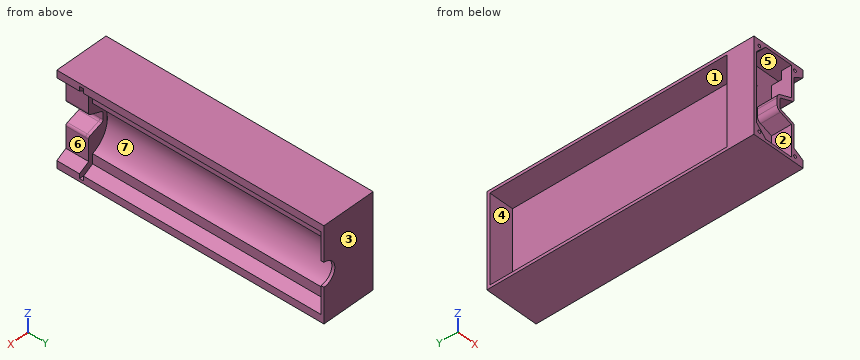
```python
from build123d import *

# Parameters (mm, degrees)
EXTRUDE_1_DEPTH     = 96
EXTRUDE_2_DEPTH     = 1.2
SKETCH_3_R          = 1.6
SKETCH_3_R_2        = 0.6
EXTRUDE_3_DEPTH     = 1.6
SKETCH_4_R          = 0.6
SKETCH_4_R_2        = 1.6
EXTRUDE_4_DEPTH     = 1.2
FILLET_1_R          = 1
SKETCH_5_R          = 1.5
CUT_EXTRUDE_1_DEPTH = 2
SKETCH_6_R          = 1.5
CUT_EXTRUDE_2_DEPTH = 2
EXTRUDE_START       = 8
EXTRUDE_6_DEPTH     = 8
SKETCH_10_R         = 0.6
EXTRUDE_7_DEPTH     = 4


with BuildPart() as part:
    # Эскиз1 → Бобышка-Вытянуть1 (new body)
    with BuildSketch(Plane(origin=(0, 0, 0), x_dir=(1, 0, 0), z_dir=(0, 1, 0))):
        with BuildLine():
            Line((0, -18.95), (0, -15.95))
            Line((0, -15.95), (-4, -13.640598923))
            Line((-4, -13.640598923), (-4, -9.708243919))
            ThreePointArc((-4, -9.708243919), (-10.5, 0), (-4, 9.708243919))
            Line((-4, 9.708243919), (-4, 13.640598923))
            Line((-4, 13.640598923), (0, 15.95))
            Line((0, 15.95), (0, 18.95))
            Line((0, 18.95), (-21.7, 18.95))
            Line((-21.7, 18.95), (-21.7, 17.75))
            Line((-21.7, 17.75), (-11.7, 17.75))
            Line((-11.7, 17.75), (-11.7, -17.75))
            Line((-11.7, -17.75), (-21.7, -17.75))
            Line((-21.7, -17.75), (-21.7, -18.95))
            Line((-21.7, -18.95), (0, -18.95))
        make_face()
    extrude(amount=EXTRUDE_1_DEPTH)

    # Эскиз2 → Бобышка-Вытянуть2 (add)
    with BuildSketch(Plane(origin=(0, 96, 0), x_dir=(1, 0, 0), z_dir=(0, 1, 0))):
        with BuildLine():
            Line((0, -4.8), (0, -18.95))
            Line((0, -18.95), (-21.7, -18.95))
            Line((-21.7, -18.95), (-21.7, 18.95))
            Line((-21.7, 18.95), (0, 18.95))
            Line((0, 18.95), (0, 4.8))
            ThreePointArc((0, 4.8), (-4.8, 0), (0, -4.8))
        make_face()
    extrude(amount=EXTRUDE_2_DEPTH)

    # Эскиз3 → Бобышка-Вытянуть3 (add)
    with BuildSketch(Plane.XZ):
        Polygon((0, -18.95), (0, -17.75), (-7, -17.75), (-12, -9.089745962), (-12, 9.089745962), (-7, 17.75), (0, 17.75), (0, 18.95), (-21.7, 18.95), (-21.7, -18.95), align=None)
        with Locations(Location((-17.7, 2.45, 0), (0, 0, 270))):
            Circle(SKETCH_3_R, mode=Mode.SUBTRACT)
        with Locations(Location((-17.7, -2.05, 0), (0, 0, 270))):
            Circle(SKETCH_3_R_2, mode=Mode.SUBTRACT)
        with Locations(Location((-17.7, 6.95, 0), (0, 0, 270))):
            Circle(SKETCH_3_R_2, mode=Mode.SUBTRACT)
    extrude(amount=EXTRUDE_3_DEPTH)

    # Эскиз4 → Бобышка-Вытянуть4 (add)
    with BuildSketch(Plane.XZ.offset(1.6)):
        Polygon((0, -17.75), (0, -18.95), (-21.7, -18.95), (-21.7, 18.95), (0, 18.95), (0, 17.75), (0, 15.95), (-4, 13.640598923), (-4, 9.708243919), (-4, 4.295838364), (-10.307764064, 2), (-10.307764064, -2), (-4, -4.295838364), (-4, -9.708243919), (-4, -13.640598923), (0, -15.95), align=None)
        with Locations(Location((-17.7, 6.95, 0), (0, 0, 270))):
            Circle(SKETCH_4_R, mode=Mode.SUBTRACT)
        with Locations(Location((-17.7, 2.45, 0), (0, 0, 270))):
            Circle(SKETCH_4_R_2, mode=Mode.SUBTRACT)
        with Locations(Location((-17.7, -2.05, 0), (0, 0, 270))):
            Circle(SKETCH_4_R, mode=Mode.SUBTRACT)
    extrude(amount=EXTRUDE_4_DEPTH)

    # Скругление1
    fillet_1_edges = [part.edges().sort_by_distance(p)[0] for p in [
        (-4, -2.2, -4.295838364),
        (-10.307764064, -2.2, -2),
        (-10.307764064, -2.2, 2),
        (-4, -2.2, 4.295838364),
    ]]
    fillet(fillet_1_edges, radius=FILLET_1_R)

    # Эскиз5 → Вырез-Вытянуть1 (cut)
    with BuildSketch(Plane.XZ.offset(2.8)):
        with Locations(Location((-13.2, 10.25, 0), (0, 0, 270))):
            Circle(SKETCH_5_R)
    extrude(amount=-CUT_EXTRUDE_1_DEPTH, mode=Mode.SUBTRACT)

    # Эскиз6 → Вырез-Вытянуть2 (cut)
    with BuildSketch(Plane.XZ.offset(2.8)):
        with Locations(Location((-13.2, -10.25, 0), (0, 0, 90))):
            Circle(SKETCH_6_R)
    extrude(amount=-CUT_EXTRUDE_2_DEPTH, mode=Mode.SUBTRACT)

    # Эскиз9 → Бобышка-Вытянуть6 (add)
    with BuildSketch(Plane.XZ.offset(2.8).offset(EXTRUDE_START)):
        with BuildLine():
            Line((-9.649784207, 2.239485083), (-4.657979857, 4.056353282))
            ThreePointArc((-4.657979857, 4.056353282), (-4.180847956, 4.422469466), (-4, 4.996045902))
            Line((-4, 4.996045902), (-4, 13.640598923))
            Line((-4, 13.640598923), (0, 15.95))
            Line((0, 15.95), (0, 18.95))
            Line((0, 18.95), (-21.7, 18.95))
            Line((-21.7, 18.95), (-21.7, -18.95))
            Line((-21.7, -18.95), (0, -18.95))
            Line((0, -18.95), (0, -15.95))
            Line((0, -15.95), (-4, -13.640598923))
            Line((-4, -13.640598923), (-4, -4.996045902))
            ThreePointArc((-4, -4.996045902), (-4.180847956, -4.422469466), (-4.657979857, -4.056353282))
            Line((-4.657979857, -4.056353282), (-9.649784207, -2.239485083))
            ThreePointArc((-9.649784207, -2.239485083), (-10.126916108, -1.873368898), (-10.307764064, -1.299792462))
            Line((-10.307764064, -1.299792462), (-10.307764064, 1.299792462))
            ThreePointArc((-10.307764064, 1.299792462), (-10.126916108, 1.873368898), (-9.649784207, 2.239485083))
        make_face()
        with BuildLine():
            Line((-1.2, 16.642820323), (-1.2, 17.75))
            Line((-1.2, 17.75), (-20.5, 17.75))
            Line((-20.5, 17.75), (-20.5, -17.75))
            Line((-20.5, -17.75), (-1.2, -17.75))
            Line((-1.2, -17.75), (-1.2, -16.642820323))
            Line((-1.2, -16.642820323), (-5.2, -14.333419246))
            Line((-5.2, -14.333419246), (-5.2, -5.13608741))
            Line((-5.2, -5.13608741), (-10.060208379, -3.367116228))
            ThreePointArc((-10.060208379, -3.367116228), (-11.109898561, -2.561660622), (-11.507764064, -1.299792462))
            Line((-11.507764064, -1.299792462), (-11.507764064, 1.299792462))
            ThreePointArc((-11.507764064, 1.299792462), (-11.109898561, 2.561660622), (-10.060208379, 3.367116228))
            Line((-10.060208379, 3.367116228), (-5.2, 5.13608741))
            Line((-5.2, 5.13608741), (-5.2, 14.333419246))
            Line((-5.2, 14.333419246), (-1.2, 16.642820323))
        make_face(mode=Mode.SUBTRACT)
    extrude(amount=-EXTRUDE_6_DEPTH)

    # Эскиз10 → Бобышка-Вытянуть7 (add)
    # profile 1 of 4: a face of its own
    with BuildSketch(Plane.XZ.offset(10.8)):
        Polygon((-1.2, 17.75), (-1.2, 16.642820323), (-5.2, 14.333419246), (-5.2, 17.75), align=None)
        with Locations(Location((-3.6, 16.55, 0), (0, 0, 270))):
            Circle(SKETCH_10_R, mode=Mode.SUBTRACT)
    # profile 2 of 4: a face of its own
    with BuildSketch(Plane.XZ.offset(10.8)):
        Polygon((-16.5, 17.75), (-20.5, 13.75), (-20.5, 17.75), align=None)
        with Locations(Location((-19.3, 16.55, 0), (0, 0, 270))):
            Circle(SKETCH_10_R, mode=Mode.SUBTRACT)
    # profile 3 of 4: a face of its own
    with BuildSketch(Plane.XZ.offset(10.8)):
        Polygon((-20.5, -13.75), (-20.5, -17.75), (-16.5, -17.75), align=None)
        with Locations(Location((-19.3, -16.55, 0), (0, 0, 90))):
            Circle(SKETCH_10_R, mode=Mode.SUBTRACT)
    # profile 4 of 4: a face of its own
    with BuildSketch(Plane.XZ.offset(10.8)):
        Polygon((-5.2, -14.333419246), (-5.2, -17.75), (-1.2, -17.75), (-1.2, -16.642820323), align=None)
        with Locations(Location((-3.6, -16.55, 0), (0, 0, 90))):
            Circle(SKETCH_10_R, mode=Mode.SUBTRACT)
    extrude(amount=-EXTRUDE_7_DEPTH)


solid = part.part
```
The listing builds one solid part. Answer for the finished solid, in the listing's coordinates (mm). Face numbers are marked on the shaded views. A direction names the side the tool comes from. Coordinates: 2 decimals unless noted, no trailing zeros. Loops run counter-clockwise (first coordinate to the right, second up) from the corner with the lowest first, then second, coordinate; pieces in that order, holes last. Notation, with made-up numbers: (8, 89.25) -> (27, 89.25) arc R24 cw to (27, 113.25) -> close; hole circle Ø6 at (-40, -32.75). An arc over 180 degrees is marked (long way). Return JSON: item names as keys, results as strings. Group by question number.
(1) Determine the mould class of the marked faces 1, 2 and 3 for opening direction Y: released by +Y, released by -Y, zero draft, split by the parting line, or undercut.
(2) Which of the six approach directions +Z, -Z, +X, -X, +Y, -Y give full straight-line access (tool end or side, diameter ignored) to the marked faces 4, 5, 6 and 7?
(3) Find the intervals of material crossed by probe 1 along Y at (x, z) = (-4.5, -15); probe 2 along Y at (x, z) = (-7, -5); probe 3 along Y at (x, z) = (-18, 0), in increasing order. Write a range as from..to.
(4) Given pin 1 Ø1.1 at (x, z) = (-19.3, -16.55) entering from -Y; pin 2 Ø0.5 at (y, z) = (-1, -2) entering from +X; pin 3 Ø1.3 at (y, z) = (-4, 0.5) entering from +X, each flat-ended and moving along its own axis, determine where each tip first touches the part or whether it passes through.
(5) A cutting plane is placed at A-A on y = 5. Write down the section's boundary in (x, z), and give its area (3 significant figures).
The answers:
{
 "1": {"face 1": "undercut", "face 2": "zero draft", "face 3": "released by +Y"},
 "2": {"face 4": "-X", "face 5": "none", "face 6": "+X, -Y", "face 7": "+X"},
 "3": {"probe 1": "y = -10.8..-6.8, -2.8..-1.6, 0..97.2", "probe 2": "y = -2.8..-1.6, 96..97.2", "probe 3": "y = -2.8..0, 96..97.2"},
 "4": {"pin 1": "stops at y = -2.8", "pin 2": "stops at x = -12", "pin 3": "stops at x = -10.31"},
 "5": {"outline": "(-21.7, -18.95) -> (0, -18.95) -> (0, -15.95) -> (-4, -13.64) -> (-4, -9.71) arc R10.5 cw to (-4, 9.71) -> (-4, 13.64) -> (0, 15.95) -> (0, 18.95) -> (-21.7, 18.95) -> (-21.7, 17.75) -> (-11.7, 17.75) -> (-11.7, -17.75) -> (-21.7, -17.75) -> close", "area": "258 mm^2"}
}
